from build123d import *

# Parameters (mm, degrees)
F0_R     = 3.302
F1_DEPTH = 5.08
F3_DEPTH = 5.08
F4_W     = 6.096
F4_H     = 19.05
F5_DEPTH = 5.08
F6_R     = 0.635
F7_W     = 2.286
F7_H     = 10.668
F8_DEPTH = 25.4
F11_D    = 1.27


with BuildPart() as f1:
    # F0 (on Top) → F1 (new body)
    with BuildSketch(Plane.XY):
        Circle(F0_R)
    extrude(amount=F1_DEPTH)

    # F2 (on face) → F3 (join, through all)
    with BuildSketch(Plane(origin=(0, 0, 0), x_dir=(1, 0, 0), z_dir=(0, 0, -1))):
        with BuildLine():
            ThreePointArc((2.2225, -2.442068), (0, -3.302), (-2.2225, -2.442068))
            Line((-2.2225, -2.442068), (-2.2225, -4.474068))
            Line((-2.2225, -4.474068), (2.2225, -4.474068))
            Line((2.2225, -4.474068), (2.2225, -2.442068))
        make_face()
    extrude(amount=-F3_DEPTH)

    # F4 (on Top) → F5 (join, through all)
    with BuildSketch(Plane.XY):
        with Locations((0, 13.999068)):
            Rectangle(F4_W, F4_H)
    extrude(amount=F5_DEPTH)

    # F6
    f6_edges = [f1.edges().sort_by_distance(p)[0] for p in [
        (3.048, 4.474068, 2.54),
        (-3.048, 4.474068, 2.54),
    ]]
    fillet(f6_edges, radius=F6_R)

    # F7 (on face) → F8 (cut)
    with BuildSketch(Plane.XY.offset(5.08)):
        with Locations((0, 12.7)):
            Rectangle(F7_W, F7_H)
    extrude(amount=-F8_DEPTH, mode=Mode.SUBTRACT)

    # F9: F1 across face


with BuildPart() as f1_1:
    add(f1.part)
    add(f1.part.mirror(Plane(origin=(0, 23.524068, 2.54), x_dir=(-1, 0, 0), z_dir=(0, 1, 0))))

    # F11 (through all)
    with Locations(Plane.YZ.offset(3.048)):
        with Locations((12.729068, 2.622667), (23.524068, 2.622667), (34.319068, 2.622667)):
            Hole(F11_D / 2)


solid = f1_1.part
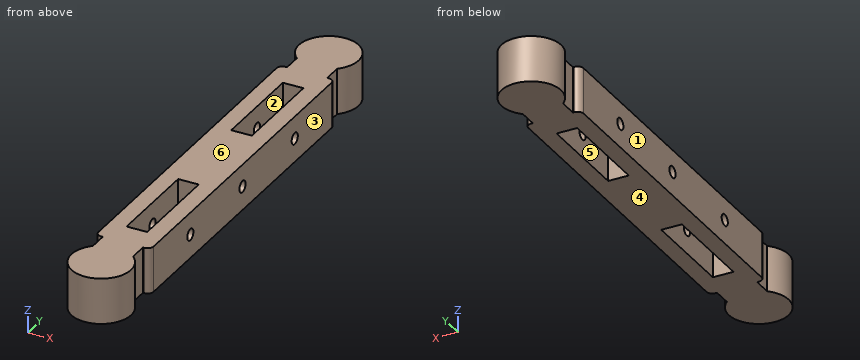
Build history of the part. All positions in model axes, mm. Face numbers are marked on the shaded views. A direction names the side the tool comes from. Coordinates: 2 decimals unless noted, no trailing zeros. Order: outer loops, then holes, each group sorted by start corner. A loop starts at its lowest first (then second) coordinate and runs counter-clockwise, first axis right, second up. Notation, with made-up numbers: (60, 82.25) - (114, 82.25) arc R22 ccw to (114, 102.25) - close; hole circle Ø3 at (7.5, 80.5). An arc over 180 degrees is marked (long way). Write each question's results on one line, items separated by ' | '. Start each with the question number.
Item 1: Band-saw the part on D-D on y = 23.5. Write the cut outline in (x, z), and give its area (3 significant figures).
Item 2: Band-saw the part on C-C on x = 0. Write the cut outline in (y, z) (3 decimals), and give its area (3 significant figures).
Item 3: Band-saw the part on A-A on y = 38.5. Write the cut outline in (x, z).
Item 4: Mould opens along Y. For the marked faces 5 and 6 say: released by +Y, released by -Y, zero draft, split by the parting line, or undercut.
Item 5: Band-saw the part on B-B on z = 1.35. State how many separate pieces and enclosed holes the cut face has, and give its area (3 significant figures).
Item 6: Flat gauge pins, fed straight in: pin 1 (1.7 mm diameter, centred on y = 12.73, z = 2.62, fed in from +X); pin 2 (1.5 mm diameter, centred on y = 23.52, z = 2.62, fed in from -X); pin 3 (1.6 mm diameter, centred on y = 44, z = 2.5, fed in from +X). Where does each tip first touch, or does it go through?
Item 7: Tool access for the marked faces 1, 2, 3 and 4: list every direction of +Z, -Z, +X, -X, +Y, -Y with a clear straight run to the whole face (end or side of a thin tool).
Item 8: Wall check: probe 1 along Y at (x, z) = (-0.25, 1.9); probe 2 along X at (y, z) = (32, 2.6); probe 3 along Y at (x, z) = (1, 3.1). Give the ranges that are in metal, low to high. Write a range as [from, to].
Numbers:
1) outline: (-3.05, 0) - (3.05, 0) - (3.05, 1.99) - (-3.05, 1.99) - close; (-3.05, 3.26) - (3.05, 3.26) - (3.05, 5.08) - (-3.05, 5.08) - close | area: 23.2 mm^2
2) outline: (-3.302, 0) - (7.366, 0) - (7.366, 5.08) - (-3.302, 5.08) - close; (18.034, 0) - (29.014, 0) - (29.014, 5.08) - (18.034, 5.08) - close; (39.682, 0) - (50.35, 0) - (50.35, 5.08) - (39.682, 5.08) - close; hole circle Ø1.27 at (23.524, 2.623) | area: 163 mm^2
3) outline: (-3.05, 0) - (-1.14, 0) - (-1.14, 5.08) - (-3.05, 5.08) - close; (1.14, 0) - (3.05, 0) - (3.05, 5.08) - (1.14, 5.08) - close
4) face 5: undercut | face 6: zero draft
5) separate pieces: 1 | enclosed holes: 2 | area: 264 mm^2
6) pin 1: x = 3.05 | pin 2: x = -3.05 | pin 3: x = 2.42
7) face 1: +Z, -Z, -X | face 2: +Z, -Z | face 3: +Z, -Z, +X | face 4: -Z, +X, -X, +Y, -Y
8) probe 1: [-3.29, 7.37], [18.03, 29.01], [39.68, 50.34] | probe 2: [-3.05, -1.14], [1.14, 3.05] | probe 3: [-3.15, 7.37], [18.03, 23.11], [23.94, 29.01], [39.68, 50.2]
